from build123d import *

# Parameters (mm, degrees)
SKETCH1_R            = 35
BOSS_EXTRUDE1_DEPTH  = 6.8
M3_CLEARANCE_HOLE1_D = 3.4
CIRPATTERN1_COUNT    = 6
SKETCH5_R            = 20.8
CUT_EXTRUDE1_DEPTH   = 3.8
SKETCH6_R            = 19.95
SKETCH6_R_2          = 17.5
CUT_EXTRUDE2_DEPTH   = 1.5
SKETCH7_R            = 42.836472813
SKETCH7_R_2          = 24.95
CUT_EXTRUDE3_DEPTH   = 2
SKETCH11_R           = 16.635
BOSS_EXTRUDE5_DEPTH  = 20.7
BOSS_EXTRUDE5_DRAFT  = -11.13
SKETCH12_R           = 17.08
CUT_EXTRUDE5_DEPTH   = 28
CUT_EXTRUDE5_DRAFT   = -11.13


with BuildPart() as part:
    # Sketch1 → Boss-Extrude1 (new body)
    with BuildSketch(Plane.XY):
        Circle(SKETCH1_R)
    extrude(amount=-BOSS_EXTRUDE1_DEPTH)

    # M3 Clearance Hole1 (through all)
    with Locations(Plane.XY):
        with Locations((-28.5, 0)):
            m3_clearance_hole1 = Hole(M3_CLEARANCE_HOLE1_D / 2)

    # CirPattern1: M3 Clearance Hole1 ×6 about axis
    cirpattern1_axis = Axis((0, 0, 0), (0, 0, 1))
    for i in range(1, CIRPATTERN1_COUNT):
        add(m3_clearance_hole1.rotate(cirpattern1_axis, i * 360 / CIRPATTERN1_COUNT), mode=Mode.SUBTRACT)

    # Sketch5 → Cut-Extrude1 (cut)
    with BuildSketch(Plane.XY):
        Circle(SKETCH5_R)
    extrude(amount=-CUT_EXTRUDE1_DEPTH, mode=Mode.SUBTRACT)

    # Sketch6 → Cut-Extrude2 (cut)
    with BuildSketch(Plane.XY.offset(-3.8)):
        Circle(SKETCH6_R)
        Circle(SKETCH6_R_2, mode=Mode.SUBTRACT)
    extrude(amount=-CUT_EXTRUDE2_DEPTH, mode=Mode.SUBTRACT)

    # Sketch7 → Cut-Extrude3 (cut)
    with BuildSketch(Plane(origin=(0, 0, -6.8), x_dir=(-1, 0, 0), z_dir=(0, 0, -1))):
        Circle(SKETCH7_R)
        Circle(SKETCH7_R_2, mode=Mode.SUBTRACT)
    extrude(amount=-CUT_EXTRUDE3_DEPTH, mode=Mode.SUBTRACT)


with BuildPart() as boss_extrude5_tool:
    # Sketch11 → Boss-Extrude5 (with draft: the straight prism first)
    with BuildSketch(Plane.XY.offset(-6.8)):
        Circle(SKETCH11_R)
    extrude(amount=-BOSS_EXTRUDE5_DEPTH)
    # Boss-Extrude5: the draft: its side faces are tilted about the plane it starts from
    boss_extrude5_sides = [boss_extrude5_tool.faces().sort_by_distance(p)[0] for p in [
        (-16.635, 0, -17.15),
    ]]
    draft(boss_extrude5_sides, Plane.XY.offset(-6.8), BOSS_EXTRUDE5_DRAFT)


with BuildPart() as part_1:
    add(part.part)

    # Boss-Extrude5: add boss_extrude5_tool
    add(boss_extrude5_tool.part)


with BuildPart() as cut_extrude5_tool:
    # Sketch12 → Cut-Extrude5 (with draft: the straight prism first)
    with BuildSketch(Plane.XY.offset(-3.8)):
        Circle(SKETCH12_R)
    extrude(amount=-CUT_EXTRUDE5_DEPTH)
    # Cut-Extrude5: the draft: its side faces are tilted about the plane it starts from
    cut_extrude5_sides = [cut_extrude5_tool.faces().sort_by_distance(p)[0] for p in [
        (-17.08, 0, -17.8),
    ]]
    draft(cut_extrude5_sides, Plane.XY.offset(-3.8), CUT_EXTRUDE5_DRAFT)


with BuildPart() as part_2:
    add(part_1.part)

    # Cut-Extrude5: cut by cut_extrude5_tool
    add(cut_extrude5_tool.part, mode=Mode.SUBTRACT)


solid = part_2.part
The listing builds one solid part. Answer for the finished solid, in the listing's coordinates (mm). A direction names the side the tool comes from. Give positions to 0.01 mm unless a question says otherwise; leave off trailing zeros. Loops run counter-clockwise (first coordinate to the right, second up) from the corner with the lowest first, then second, coordinate; pieces in that order, holes last.
Item 1: A cutting plane is placed at A-A (x = -28.5). Give the vertices of the cut face in (y, z).
Derived:
outline: (-20.32, -4.8) - (-1.7, -4.8) - (-1.7, 0) - (-20.32, 0) - close; (1.7, -4.8) - (20.32, -4.8) - (20.32, 0) - (1.7, 0) - close
Item 2: A cutting plane is placed at B-B (y = 0). Give the number of separate pieces and of enclosed holes in the cut face, then the cut area to 3 significant figures.
Derived:
separate pieces: 4
enclosed holes: 0
area: 143 mm2
Item 3: Find the intervals of material crossed by line 1 along X through (y, z) = (-14, -4.25); line 2 along Y through (x, z) = (-14.25, -2.85); line 3 along Z through (x, y) = (-27, 8.5), in increasing order.
Derived:
line 1: x = -32.08 to -14.21, -10.5 to -9.63, 9.63 to 10.5, 14.21 to 32.08
line 2: y = -31.97 to -26.38, -22.98 to -15.15, 15.15 to 22.98, 26.38 to 31.97
line 3: z = -4.8 to 0
Item 4: A cutting plane is placed at C-C (z = -25.5). Give the vertices of the cut face in (x, y), then the cut area to 3 significant figures.
Derived:
outline: circle Ø25.91 at (0, 0); hole circle Ø25.62 at (0, 0)
area: 11.8 mm2
Item 5: A tool of negligible diameter and unlimited length cuts with its end or side. For faces 5 (the flat face through (0, -18, -5.3)), 6 (the cylindrical face through (-14.619, -23.022, -2.434)), 7 (the flat face through (-23, 11, -4.8)), from which of +Z, -Z, +X, -X, +Y, -Y can it reach the whole face along a straight path? Write none if from no direction.
Derived:
face 5: +Z
face 6: +Z, -Z
face 7: -Z
Item 6: Determine the mould class of faces 1 (the cylindrical face through (-13.887, -10.648, -4.54)), 2 (the cylindrical face through (-23.8, 7.49, -5.81)), 3 (the cylindrical face through (-13.336, 23.248, -2.434)), 4 (the flat face through (5.2, -16.3, -6.8)) for opening direction Y: +Y half, -Y half, draft (parallel to the pull), parting line (faces both ways), or undercut.
Derived:
face 1: undercut
face 2: parting line
face 3: undercut
face 4: draft
Item 7: Each of these flat-tipped pins is pushed along its axis until it touches: pin 1 Ø8 at (x, z) = (18, -6.5) entering from -Y; pin 2 Ø3 at (x, y) = (-14.25, -24.68) entering from -Z; pin 3 Ø12 at (y, z) = (11.5, -7.5) entering from +X; pin 4 Ø5 at (y, z) = (-17, -7) entering from +X. Where does it stop, or does it pass through?
Derived:
pin 1: stops at y = -31.91
pin 2: passes through
pin 3: stops at x = 34.46
pin 4: stops at x = 31.22
